from build123d import *

# Parameters (mm, degrees)
SKETCH_1_W      = 400
SKETCH_1_H      = 100
EXTRUDE_1_DEPTH = 200
FILLET_1_R      = 20
SHELL_1_T       = -3


with BuildPart() as part:
    # 草圖1 → 伸長1 (new body)
    with BuildSketch(Plane.XY):
        with Locations((0, 50)):
            Rectangle(SKETCH_1_W, SKETCH_1_H)
    extrude(amount=EXTRUDE_1_DEPTH)

    # 圓角1
    fillet_1_edges = [part.edges().sort_by_distance(p)[0] for p in [
        (200, 0, 100),
        (-200, 0, 100),
    ]]
    fillet(fillet_1_edges, radius=FILLET_1_R)

    # 薄殼1
    shell_1_openings = [part.faces().sort_by_distance(p)[0] for p in [
        (0, 50.196270167, 200),
        (0, 50.196270167, 0),
        (0, 100, 100),
    ]]
    offset(amount=SHELL_1_T, openings=shell_1_openings, kind=Kind.INTERSECTION)


solid = part.part
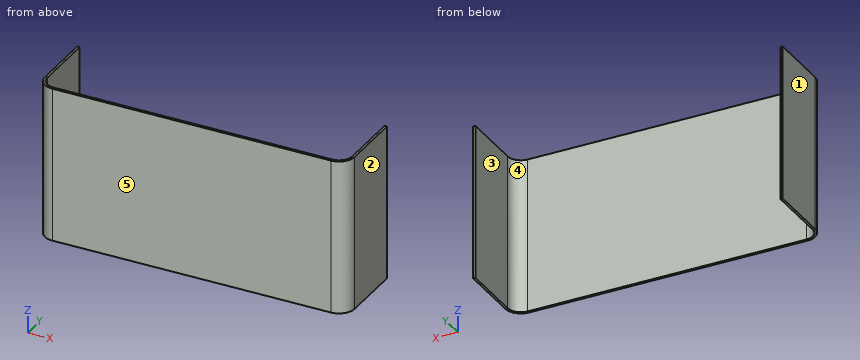
Source: CAD feature listing. Evaluate the final solid. Frame: model axes, mm. Face numbers are marked on the shaded views. A direction names the side the tool comes from. Give positions to 0.01 mm unless a question says otherwise; leave off trailing zeros. Write each loop counter-clockwise with the first axis right and the second up, starting at its lowest first coordinate (ties: lowest second). Pieces come first, ordered by that corner, then holes. Notation, with made-up numbers: (82, 50) - (115, 50) arc R27 ccw to (115, 66) - close; hole circle Ø9 at (-34, 59.25). An arc over 180 degrees is marked (long way). Write item = value, one per line. Start each with the question number.
Q1. Draft query along X for the marked faces 1, 2 and 3. Return one class per face: +X half, -X half, draft (parallel to the pull), parting line (faces both ways), or undercut.
Q2. Cut plane B-B, the plane z = 158. Return loops of the section in (x, y).
Q3. Material intervals for probe 1 along X at (y, z) = (72.5, 152); probe 2 along Y at (x, z) = (-176, 192.5); probe 3 along X at (y, z) = (16, 16), sorted ascending.
Q4. Reachability of the marked faces 4 and 5 from +Z, -Z, +X, -X, +Y, -Y: full face, straight path, thin tool, end or side. Return the list, or none.
Q5. Cut plane D-D, the plane y = 7. Return loops of the section in (x, z).
Q6. Cut plane C-C, the plane x = 126.5. Return loops of the section in (y, z).
Q7. Pin query (flat end, axial travel): pin 1 Ø12 at (x, z) = (63.5, 156.5) entering from +Y; pin 2 Ø10 at (y, z) = (13.5, 45.5) entering from +X; pin 3 Ø4 at (y, z) = (17.5, 154.5) entering from +X. Return the tip coordinate at first contact, or that it passes through.
Q8. Cut plane A-A, the plane y = 50. Return loops of the section in (x, z), then the cut area to 3 significant figures.
Computed values:
q1.face_1 = -X half
q1.face_2 = +X half
q1.face_3 = undercut
q2.outline = (-200, 20) arc R20 ccw to (-180, 0) - (180, 0) arc R20 ccw to (200, 20) - (200, 100) - (197, 100) - (197, 20) arc R17 cw to (180, 3) - (-180, 3) arc R17 cw to (-197, 20) - (-197, 100) - (-200, 100) - close
q3.probe_1 = -200 to -197, 197 to 200
q3.probe_2 = 0 to 3
q3.probe_3 = -199.6 to -196.52, 196.52 to 199.6
q4.face_4 = +Z, -Z, +Y
q4.face_5 = +Z, -Z, +X, -X, -Y
q5.outline = (-195.2, 0) - (-190.95, 0) - (-190.95, 200) - (-195.2, 200) - close; (190.95, 0) - (195.2, 0) - (195.2, 200) - (190.95, 200) - close
q6.outline = (0, 0) - (3, 0) - (3, 200) - (0, 200) - close
q7.pin_1 = 3
q7.pin_2 = 199.94
q7.pin_3 = 199.99
q8.outline = (-200, 0) - (-197, 0) - (-197, 200) - (-200, 200) - close; (197, 0) - (200, 0) - (200, 200) - (197, 200) - close
q8.area = 1,200 mm²
